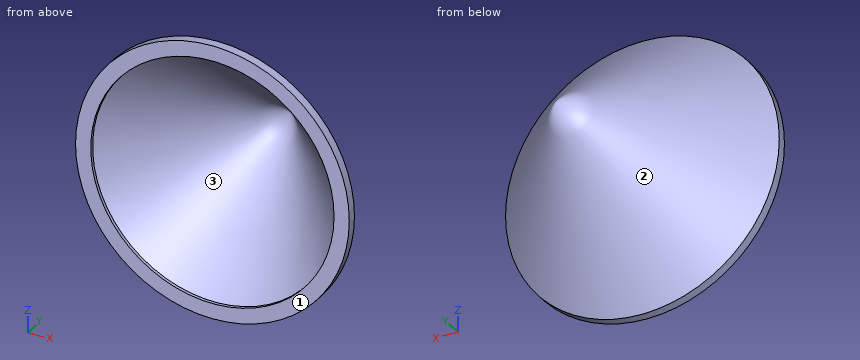
Autodesk Fusion 360 part; units mm, degrees
sketch "Sketch1" plane through (0, 0, 0) normal (0, 1, 0) x (1, 0, 0)
  circle A0 centre (0, 0) radius 45
  dimension "d1" = 90
extrude "Extrude1" add sketch "Sketch1" along normal blind 100 makes body 1
sketch "Sketch2" plane through (0, 100, 0) normal (0, 1, 0) x (-1, 0, 0)
  circle A0 centre (0, 0) radius 45
  circle A1 centre (0, 0) radius 42.5
  dimension "d4" = 85
extrude "Extrude2" cut sketch "Sketch2" against normal blind 110 contours A1 bodies 1
sketch "Sketch3" plane through (0, 0, 0) normal (0, 0, 1) x (1, 0, 0)
extrude "Extrude3" add sketch "Sketch1" along normal blind 3 separate body makes body 2
sketch "Sketch4" plane through (0, 0, 0) normal (0, 0, 1) x (1, 0, 0)
  line L0 (0, 3) -> (0, 53)
  line L1 (0, 53) -> (45, 3)
  line L2 (45, 3) -> (0, 3)
  dimension "d9" = 50
revolve "Revolve1" add sketch "Sketch4" angle 360 about axis through (0, 3, 0) along (0, 1, 0) bodies 2
shell "Shell1" thickness 5 removed faces 1 at (4.1569, 0, 25.5535) on bodies 2
hidden bodies 1
Build history of the part. All positions in model axes, mm. Face numbers are marked on the shaded views. Give positions to 0.01 mm unless a question says otherwise; leave off trailing zeros. Loops run counter-clockwise (first coordinate to the right, second up) from the corner with the lowest first, then second, coordinate; pieces in that order, holes last. Notation, with made-up numbers: (71, 55.25) - (127, 55.25) arc R29 cw to (127, 90.25) - close; hole circle Ø11 at (-8, 31.5). An arc over 180 degrees is marked (long way). Use a Markdown table: item, result.
(1) Band-saw the part on A-A (y = 36). Give the cut face in (x, z), and give its area (3 significant figures).
Taken from the geometry:
| item | result |
|---|---|
| outline | circle Ø30.6 at (0, 0); hole circle Ø17.15 at (0, 0) |
| area | 505 mm2 |
(2) Band-saw the part on B-B (y = 26). Give the cut face in (x, z).
Taken from the geometry:
| item | result |
|---|---|
| outline | circle Ø48.6 at (0, 0); hole circle Ø35.15 at (0, 0) |
(3) Wall check: line 1 along Z through (x, y) = (0, 0.55); line 2 along Z through (x, y) = (-19.5, 11); line 3 along X through (y, z) = (29.5, 2.5). Give the ranges that are in metal, low to high.
Taken from the geometry:
| item | result |
|---|---|
| line 1 | -45 to -40, 40 to 45 |
| line 2 | -32.38 to -24.19, 24.19 to 32.38 |
| line 3 | -21 to -14.2, 14.2 to 21 |
(4) Pull direction Z, two halves, no side cores. Call the marked faces 1, 2 and 3: +Z half, -Z half, draft (parallel to the pull), parting line (faces both ways), or undercut.
Taken from the geometry:
| item | result |
|---|---|
| face 1 | draft |
| face 2 | parting line |
| face 3 | undercut |
(5) Drop flat-ended pins along their axis: pin 1 Ø4 at (y, z) = (31.5, 7) entering from +X; pin 2 Ø1 at (x, y) = (-20.5, 6.5) entering from +Z; pin 3 Ø5 at (x, z) = (-8, -27) entering from +Y. Give the stop position or say it passes through.
Taken from the geometry:
| item | result |
|---|---|
| pin 1 | x = 20.07 |
| pin 2 | z = 37.07 |
| pin 3 | y = 24.49 |
